```python
from build123d import *

# Parameters (mm, degrees)
BOSS_EXTRUDE1_DEPTH = 2.5
FILLET1_R           = 1
FILLET2_R           = 0.5


with BuildPart() as part:
    # Sketch3 → Boss-Extrude1 (new, symmetric)
    with BuildSketch(Plane.XY):
        Polygon((-22.35, 376.5), (-62.3, 20), (-62.3, 0), (62.3, 0), (62.3, 20), (22.35, 376.5), (22.35, 167.1), (17.35, 167.1), (17.35, 314.2), (-17.35, 314.2), (-17.35, 167.1), (-22.35, 167.1), align=None)
    extrude(amount=BOSS_EXTRUDE1_DEPTH, both=True)

    # Fillet1
    fillet1_edges = [part.edges().sort_by_distance(p)[0] for p in [
        (-17.35, 314.2, 0),
        (17.35, 314.2, 0),
        (62.3, 0, 0),
        (-62.3, 0, 0),
    ]]
    fillet(fillet1_edges, radius=FILLET1_R)

    # Fillet2
    fillet2_edges = [part.edges().sort_by_distance(p)[0] for p in [
        (22.35, 376.5, 0),
        (-22.35, 376.5, 0),
    ]]
    fillet(fillet2_edges, radius=FILLET2_R)


solid = part.part
```
Build history of the part. All positions in model axes, mm. Give positions to 0.01 mm unless a question says otherwise; leave off trailing zeros. Order: outer loops, then holes, each group sorted by start corner. A loop starts at its lowest first (then second) coordinate and runs counter-clockwise, first axis right, second up. Notation, with made-up numbers: M -25.75,-24.5 L -11.75,-24.5 A12 cw -11.75,-17.5 Z; hole C 31.5,17.25 d3. An arc over 180 degrees is marked long. Write item = value, one per line. Start each with the question number.
(1) Slice it at C-C on y = 256.5. Write the cut outline in (x, z), plus the area to 3 significant figures.
(2) Slice it at D-D on x = -11.5. Write the cut outline in (y, z).
(3) Pin check, flat tips, straight feed: pin 1 Ø1.5 at (x, z) = (-20, 1) entering from +Y; pin 2 Ø1.5 at (y, z) = (259, -1) entering from -X; pin 3 Ø2.5 at (y, z) = (304, -1) entering from +X. Stop position of each tip, or through.
(4) Slice it at B-B on z = 0.7. Write the cut outline in (x, y).
(5) Probe L1, parallel to X at y = 192.5, z = -2.05; L2, parallel to X at y = 231, z = -0.35; L3, parallel to X at y = 29, z = 1.05. List the from-to ranges inside material, lowest first. Write a range as [from, to].
(6) Slice it at A-A on y = 330. Write the cut outline in (x, z).
Responses:
q1.outline = M -35.8,-2.5 L -22.35,-2.5 L -22.35,2.5 L -35.8,2.5 Z; M -17.35,-2.5 L 17.35,-2.5 L 17.35,2.5 L -17.35,2.5 Z; M 22.35,-2.5 L 35.8,-2.5 L 35.8,2.5 L 22.35,2.5 Z
q1.area = 308 mm2
q2.outline = M 0,-2.5 L 314.2,-2.5 L 314.2,2.5 L 0,2.5 Z
q3.pin_1 = 167.1
q3.pin_2 = -35.6
q3.pin_3 = 30.61
q4.outline = M -62.3,1 A1 ccw -61.3,0 L 61.3,0 A1 ccw 62.3,1 L 62.3,20 L 23.35,367.6 A0.5 ccw 22.35,367.55 L 22.35,167.1 L 17.35,167.1 L 17.35,313.2 A1 ccw 16.35,314.2 L -16.35,314.2 A1 ccw -17.35,313.2 L -17.35,167.1 L -22.35,167.1 L -22.35,367.55 A0.5 ccw -23.35,367.6 L -62.3,20 Z
q5.L1 = [-42.97, -22.35], [-17.35, 17.35], [22.35, 42.97]
q5.L2 = [-38.65, -22.35], [-17.35, 17.35], [22.35, 38.65]
q5.L3 = [-61.29, 61.29]
q6.outline = M -27.56,-2.5 L -22.35,-2.5 L -22.35,2.5 L -27.56,2.5 Z; M 22.35,-2.5 L 27.56,-2.5 L 27.56,2.5 L 22.35,2.5 Z
